The listing builds one solid part. Answer for the finished solid, in the listing's coordinates (mm). A direction names the side the tool comes from. Give positions to 0.01 mm unless a question says otherwise; leave off trailing zeros. Write each loop counter-clockwise with the first axis right and the second up, starting at its lowest first coordinate (ties: lowest second). Pieces come first, ordered by that corner, then holes. Notation, with made-up numbers: (65.5, -3) - (119.5, -3) arc R14 cw to (119.5, 15) - close; hole circle Ø11 at (0.25, 40.5). An arc over 180 degrees is marked (long way). One line per question, with ' | ' between items. Start each with the question number.
1. A cutting plane is placed at B-B (x = -21.9). Determine the outline of the cut face in (y, z).
2. The mould has two halves that part along Z. Classify faces 3 (the face through (-7.78, -2.028, -24.704)), 4 (the face through (-6, 0, 0)), 5 (the face through (-10.884, -2.028, 17.467)): +Z half, -Z half, draft (parallel to the pull), parting line (faces both ways), or undercut.
3. For faces 1 (the face through (-5.7, 32.04, 0.75)), 2 (the face through (0, -4, 0)), determine the directions among +Z, -Z, +X, -X, +Y, -Y from which every point of the face is accessible in a straight line to the end or side of a thin tool.
4. A cutting plane is placed at D-D (x = 10.95). Determine the outline of the cut face in (y, z), then the cut area to 3 significant figures.
5. Given P1, Ø5, axis at x = -21.9, z = 0, coming from the +Y side; P2, Ø5, axis at y = 39.5, z = 6.5, coming from the +X side; P3, Ø1.8, axis at x = -10.95, z = 18.97, coming from the +Y side; P4, Ø12, axis at y = 12.5, z = -4, coming from the -X side, each flat-ended and moving along its own axis, determine where each tip first touches the part or whether it passes through.
6. Find the intervals of material crossed by L1, parallel to X at y = -1.2, z = 0; L2, parallel to Z at x = -10.95, y = -1.05; L3, parallel to Y at x = -18, z = -9.5, in increasing order. Write a range as from..to.
7. A cutting plane is placed at C-C (x = 0). Determine the outline of the cut face in (y, z), then the cut area to 3 significant figures.
8. A cutting plane is placed at A-A (z = 0). Determine the outline of the cut face in (x, y).
```python
from build123d import *

# Parameters (mm, degrees)
CUT_EXTRUDE_1_DEPTH      = 75.609784881
CUT_EXTRUDE_1_DEPTH_BACK = 75.609784881
SKETCH_2_R               = 1.5


with BuildPart() as part:
    # Эскиз1 → Повернуть1 (revolve)
    with BuildSketch(Plane.XY, mode=Mode.PRIVATE) as revolve_1_sk:
        Polygon((5.75, 0), (25.9, 0), (25.9, -4), (0, -4), (0, 65), (5.75, 65), align=None)
    revolve(revolve_1_sk.sketch.rotate(Axis((0, 0, 0), (0, 1, 0)), 90), axis=Axis((0, 0, 0), (0, 1, 0)))

    # Эскиз2 → Вырез-Вытянуть1 (cut, two sides: drawn at the far end of the back side and taken through both)
    with BuildSketch(Plane(origin=(0, 0, 0), x_dir=(1, 0, 0), z_dir=(0, 1, 0)).offset(-CUT_EXTRUDE_1_DEPTH_BACK)):
        with Locations(Location((21.9, 0, 0), (0, 0, 270))):
            Circle(SKETCH_2_R)
        with Locations(Location((10.95, -18.965956343, 0), (0, 0, 270))):
            Circle(SKETCH_2_R)
        with Locations(Location((-10.95, -18.965956343, 0), (0, 0, 270))):
            Circle(SKETCH_2_R)
        with Locations(Location((-21.9, 0, 0), (0, 0, 270))):
            Circle(SKETCH_2_R)
        with Locations(Location((-10.95, 18.965956343, 0), (0, 0, 270))):
            Circle(SKETCH_2_R)
        with Locations(Location((10.95, 18.965956343, 0), (0, 0, 270))):
            Circle(SKETCH_2_R)
    extrude(amount=CUT_EXTRUDE_1_DEPTH + CUT_EXTRUDE_1_DEPTH_BACK, mode=Mode.SUBTRACT)


solid = part.part
```
Determined:
1) outline: (-4, -13.83) - (0, -13.83) - (0, -1.5) - (-4, -1.5) - close; (-4, 1.5) - (0, 1.5) - (0, 13.83) - (-4, 13.83) - close
2) face 3: parting line | face 4: draft | face 5: undercut
3) face 1: +Y | face 2: +Z, -Z, +X, -X, -Y
4) outline: (-4, -23.47) - (0, -23.47) - (0, -20.47) - (-4, -20.47) - close; (-4, -17.47) - (0, -17.47) - (0, 17.47) - (-4, 17.47) - close; (-4, 20.47) - (0, 20.47) - (0, 23.47) - (-4, 23.47) - close | area: 164 mm2
5) P1: y = 0 | P2: x = 4.13 | P3: through | P4: x = -5.75
6) L1: -25.9..-23.4, -20.4..20.4, 23.4..25.9 | L2: -23.47..-20.47, -17.47..17.47, 20.47..23.47 | L3: -4..0
7) outline: (-4, -25.9) - (0, -25.9) - (0, -5.75) - (65, -5.75) - (65, 5.75) - (0, 5.75) - (0, 25.9) - (-4, 25.9) - close | area: 955 mm2
8) outline: (-25.9, -4) - (-23.4, -4) - (-23.4, 0) - (-25.9, 0) - close; (-20.4, -4) - (20.4, -4) - (20.4, 0) - (5.75, 0) - (5.75, 65) - (-5.75, 65) - (-5.75, 0) - (-20.4, 0) - close; (23.4, -4) - (25.9, -4) - (25.9, 0) - (23.4, 0) - close
